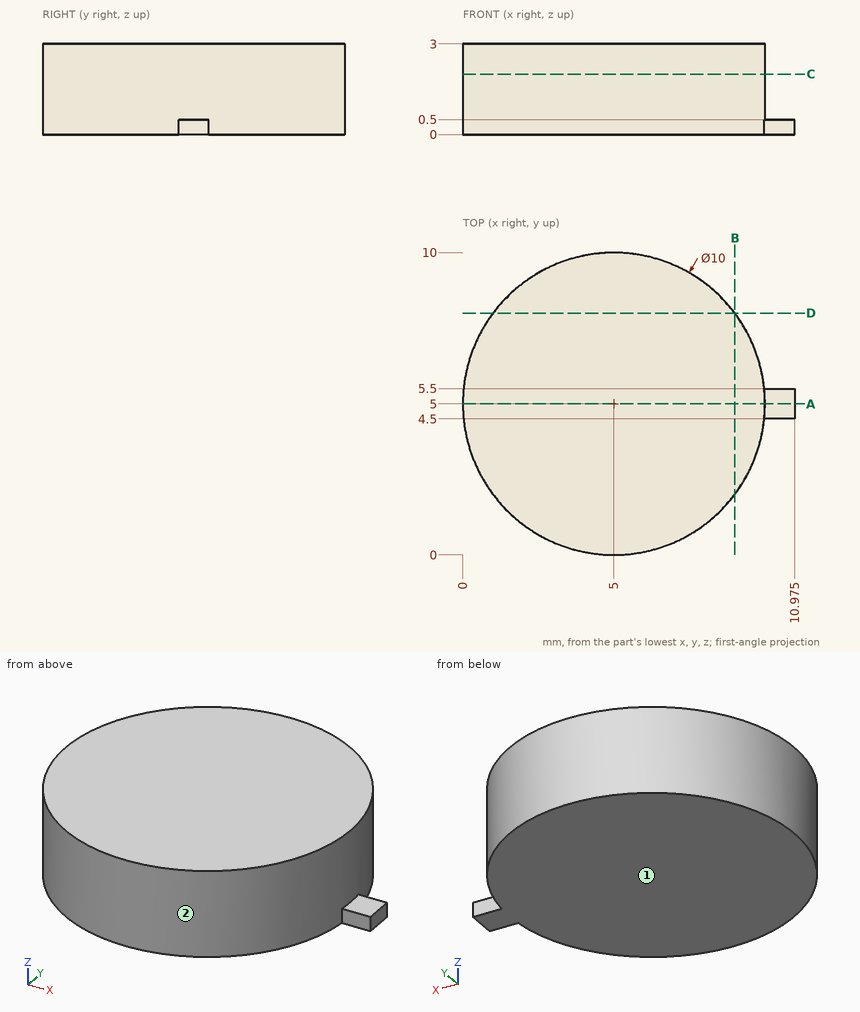
Check sheet for the drawn part. Datum: minimum x, y, z corner. Units: mm. Round coordinates to 2 decimals unless told otherwise and drop trailing zeros. Write each loop counter-clockwise with the first axis right and the second up, starting at its lowest first coordinate (ties: lowest second). Pieces come first, ordered by that corner, then holes. Notation, with made-up numbers: (-29.75, -0.5) -> (2.25, -0.5) arc R19 ccw to (2.25, 21.5) -> close; hole circle Ø5 at (77, -25.5). An arc over 180 degrees is marked (long way). One line per item, written item: value. Start each with the question number.
(1) Cross-section at C-C, the plane z = 2. Record the cut outline in (x, y).
(2) Cross-section at D-D, the plane y = 8. Record the cut outline in (x, z), and give its area (3 significant figures).
(3) Draft check along Y on the marked faces 1 and 2. Enter one of: +Y half, -Y half, draft (parallel to the pull), parting line (faces both ways), or undercut.
(4) Scan lines: line 1 (X direction, y = 4.75, z = 1.75); line 2 (Y direction, x = 8, z = 0.35); line 3 (Y direction, x = 7.25, z = 0.5) (3 decimals). Record each from-to range of solid material in increasing order. Write a range as [from, to].
(5) Go/stop test with flat-tipped pins: pin 1 Ø0.5 at (x, y) = (10.5, 5) entering from +Z; pin 2 Ø1 at (x, z) = (8.5, 1) entering from -Y; pin 3 Ø1.5 at (y, z) = (7, 2.5) entering from -X. Record where each tip stops, or that it passes through.
(6) Cross-section at A-A, the plane y = 5. Record the cut outline in (x, z) (3 decimals), and give its area (3 significant figures).
(7) Cross-section at B-B, the plane x = 9. Record the cut outline in (y, z).
Answer:
1. outline: circle Ø10 at (5, 5)
2. outline: (1, 0) -> (9, 0) -> (9, 3) -> (1, 3) -> close
2. area: 24.0 mm²
3. face 1: draft
3. face 2: parting line
4. line 1: [0.01, 9.99]
4. line 2: [1, 9]
4. line 3: [0.535, 9.465]
5. pin 1: z = 0.5
5. pin 2: y = 1
5. pin 3: x = 0.16
6. outline: (0, 0) -> (10.975, 0) -> (10.975, 0.5) -> (10, 0.5) -> (10, 3) -> (0, 3) -> close
6. area: 30.5 mm²
7. outline: (2, 0) -> (8, 0) -> (8, 3) -> (2, 3) -> close
